from build123d import *

# Parameters (mm, degrees)
ESQUISSE1_W             = 50
ESQUISSE1_H             = 100
BOSS_EXTRU_1_DEPTH      = 3
ESQUISSE3_W             = 20
ESQUISSE3_H             = 20
ESQUISSE3_H_2           = 31
ENL_V_MAT_EXTRU_2_DEPTH = 3
ESQUISSE5_W             = 10.07
ESQUISSE5_H             = 3
ENL_V_MAT_EXTRU_3_DEPTH = 3
ESQUISSE6_W             = 0.13
ESQUISSE6_H             = 3
ENL_V_MAT_EXTRU_4_DEPTH = 3


with BuildPart() as part:
    # Esquisse1 → Boss.-Extru.1 (new body)
    with BuildSketch(Plane.XY):
        with Locations((25, 50)):
            Rectangle(ESQUISSE1_W, ESQUISSE1_H)
    extrude(amount=BOSS_EXTRU_1_DEPTH)

    # Esquisse3 → Enlèv. mat.-Extru.2 (cut)
    with BuildSketch(Plane.XY.offset(3)):
        with Locations((25, 75.953744756)):
            Rectangle(ESQUISSE3_W, ESQUISSE3_H)
        with Locations((25, 32.989712488)):
            Rectangle(ESQUISSE3_W, ESQUISSE3_H_2)
    extrude(amount=-ENL_V_MAT_EXTRU_2_DEPTH, mode=Mode.SUBTRACT)

    # Esquisse5 → Enlèv. mat.-Extru.3 (cut)
    with BuildSketch(Plane.XY.offset(3)):
        with Locations((24.935, 98.5)):
            Rectangle(ESQUISSE5_W, ESQUISSE5_H)
        with Locations((5.035, 98.5)):
            Rectangle(ESQUISSE5_W, ESQUISSE5_H)
        with Locations((44.835, 98.5)):
            Rectangle(ESQUISSE5_W, ESQUISSE5_H)
        with Locations((24.935, 1.5)):
            Rectangle(ESQUISSE5_W, ESQUISSE5_H)
        with Locations((44.835, 1.5)):
            Rectangle(ESQUISSE5_W, ESQUISSE5_H)
        with Locations((5.035, 1.5)):
            Rectangle(ESQUISSE5_W, ESQUISSE5_H)
    extrude(amount=-ENL_V_MAT_EXTRU_3_DEPTH, mode=Mode.SUBTRACT)

    # Esquisse6 → Enlèv. mat.-Extru.4 (cut)
    with BuildSketch(Plane.XY.offset(3)):
        with Locations((49.935, 98.5)):
            Rectangle(ESQUISSE6_W, ESQUISSE6_H)
        with Locations((49.935, 1.5)):
            Rectangle(ESQUISSE6_W, ESQUISSE6_H)
    extrude(amount=-ENL_V_MAT_EXTRU_4_DEPTH, mode=Mode.SUBTRACT)


solid = part.part
Read the model definition and answer for the solid it produces. Units are mm, in the model's axes. A direction names the side the tool comes from. Coordinates: 2 decimals unless noted, no trailing zeros. Order: outer loops, then holes, each group sorted by start corner. A loop starts at its lowest first (then second) coordinate and runs counter-clockwise, first axis right, second up. Notation, with made-up numbers: (-39, 12) -> (8, 12) arc R28 ccw to (8, 44) -> close; hole circle Ø10 at (17.5, 1). An arc over 180 degrees is marked (long way). Answer as a JSON object with one key per item and string values.
1) A cutting plane is placed at C-C, the plane x = 31. Determine the outline of the cut face in (y, z).
Model answer:
{"outline": "(0, 0) -> (17.49, 0) -> (17.49, 3) -> (0, 3) -> close; (48.49, 0) -> (65.95, 0) -> (65.95, 3) -> (48.49, 3) -> close; (85.95, 0) -> (100, 0) -> (100, 3) -> (85.95, 3) -> close"}
2) Consider line 1 along Y through (x, z) = (34, 1.8); line 2 along Y through (x, z) = (20, 1.25); line 3 along X through (y, z) = (74, 2.2). Determine where each line is inside the solid, lowest interval first. Write a range as from..to.
Model answer:
{"line 1": "y = 0..17.49, 48.49..65.95, 85.95..100", "line 2": "y = 3..17.49, 48.49..65.95, 85.95..97", "line 3": "x = 0..15, 35..50"}
3) Each of these flat-tipped pins is pushed along its axis until it touches: pin 1 (0.9 mm diameter, centred on x = 3.5, z = 1, fed in from -Y); pin 2 (1.5 mm diameter, centred on x = 4, z = 1, fed in from +Y); pin 3 (1.5 mm diameter, centred on y = 99, z = 1.5, fed in from +X). Where does it stop, or does it pass through?
Model answer:
{"pin 1": "stops at y = 3", "pin 2": "stops at y = 97", "pin 3": "stops at x = 39.8"}
4) A cutting plane is placed at B-B, the plane y = 19. Determine the outline of the cut face in (x, z).
Model answer:
{"outline": "(0, 0) -> (15, 0) -> (15, 3) -> (0, 3) -> close; (35, 0) -> (50, 0) -> (50, 3) -> (35, 3) -> close"}
5) A tool of negligible diameter and unlimited length cuts with its end or side. For faces 1 (the face through (45, 97, 2)), 2 (the face through (19.9, 98, 2)), 3 (the face through (25, 3, 2)), 4 (the face through (25, 48.49, 2)), from which of +Z, -Z, +X, -X, +Y, -Y can it reach the whole face along a straight path? Write none if from no direction.
Model answer:
{"face 1": "+Z, -Z, +X, +Y", "face 2": "+Z, -Z, +Y", "face 3": "+Z, -Z, -Y", "face 4": "+Z, -Z"}
6) A cutting plane is placed at D-D, the plane x = 43.5. Determine the outline of the cut face in (y, z), plus the area to 3 significant figures.
Model answer:
{"outline": "(3, 0) -> (97, 0) -> (97, 3) -> (3, 3) -> close", "area": "282 mm²"}
7) A cutting plane is placed at A-A, the plane z = 2.5. Determine the outline of the cut face in (x, y).
Model answer:
{"outline": "(0, 3) -> (10.07, 3) -> (10.07, 0) -> (19.9, 0) -> (19.9, 3) -> (29.97, 3) -> (29.97, 0) -> (39.8, 0) -> (39.8, 3) -> (50, 3) -> (50, 97) -> (39.8, 97) -> (39.8, 100) -> (29.97, 100) -> (29.97, 97) -> (19.9, 97) -> (19.9, 100) -> (10.07, 100) -> (10.07, 97) -> (0, 97) -> close; hole (15, 17.49) -> (35, 17.49) -> (35, 48.49) -> (15, 48.49) -> close; hole (15, 65.95) -> (35, 65.95) -> (35, 85.95) -> (15, 85.95) -> close"}
8) The mould has two halves that part along Y. Classify faces 5 (the face through (25, 51, 0)), 6 (the face through (35, 33, 2)), 7 (the face through (35, 100, 1)), 8 (the face through (25, 65.954, 2)): released by +Y, released by -Y, zero draft, split by the parting line, or undercut.
Model answer:
{"face 5": "zero draft", "face 6": "undercut", "face 7": "released by +Y", "face 8": "undercut"}
